Design review of the part built by this model. Coordinates are the model's own, in mm. Face numbers are marked on the shaded views. A direction names the side the tool comes from. Give positions to 0.01 mm unless a question says otherwise; leave off trailing zeros. Loops run counter-clockwise (first coordinate to the right, second up) from the corner with the lowest first, then second, coordinate; pieces in that order, holes last. Notation, with made-up numbers: M 66,61 L 117,61 A25 cw 117,78 Z; hole C 41,81.25 d9. An arc over 180 degrees is marked long. Answer as CSV lines item,"result".
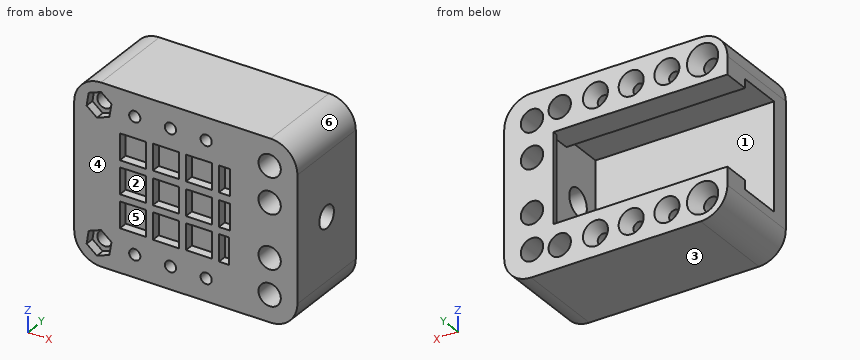
```python
from build123d import *

# Parameters (mm, degrees)
SKETCH1_W                                         = 63.5
SKETCH1_H                                         = 50.8
BOSS_EXTRUDE1_DEPTH                               = 25.4
FILLET1_R                                         = 7.62
CUT_EXTRUDE1_DEPTH                                = 50.8
SKETCH4_W                                         = 49.53
SKETCH4_H                                         = 25.4
CUT_EXTRUDE2_DEPTH                                = 13.462
CSK_FOR_2_FLAT_HEAD_MACHINE_SCREW_100_D           = 4.318
CSK_FOR_2_FLAT_HEAD_MACHINE_SCREW_100_CSINK_D     = 8.89
CSK_FOR_2_FLAT_HEAD_MACHINE_SCREW_100_CSINK_ANGLE = 60
CSK_FOR_2_FLAT_HEAD_MACHINE_SCREW_2_D             = 3.175
CSK_FOR_2_FLAT_HEAD_MACHINE_SCREW_2_CSINK_D       = 7.112
CSK_FOR_2_FLAT_HEAD_MACHINE_SCREW_2_CSINK_ANGLE   = 60
SKETCH9_R                                         = 3.175
CUT_EXTRUDE3_DEPTH                                = 12.7
F_1_4_0_25_DIAMETER_HOLE1_D                       = 6.35
F_1_4_0_25_DIAMETER_HOLE2_D                       = 6.35
CUT_EXTRUDE4_DEPTH                                = 2.54
SKETCH15_W                                        = 3.09588561
SKETCH15_H                                        = 7.430125466
SKETCH15_W_2                                      = 7.430125466
SKETCH15_H_2                                      = 7.430125465
SKETCH15_W_3                                      = 2.91808561
SKETCH15_H_3                                      = 7.607925465
CUT_EXTRUDE5_DEPTH                                = 2.54
SKETCH16_R                                        = 3.175
CUT_EXTRUDE8_DEPTH                                = 6.985
SKETCH17_R                                        = 3.81
CUT_EXTRUDE9_DEPTH                                = 6.985


with BuildPart() as part:
    # Sketch1 → Boss-Extrude1 (new body)
    with BuildSketch(Plane(origin=(0, 0, 0), x_dir=(1, 0, 0), z_dir=(0, 1, 0))):
        with Locations((31.75, 25.4)):
            Rectangle(SKETCH1_W, SKETCH1_H)
    extrude(amount=BOSS_EXTRUDE1_DEPTH)

    # Fillet1
    fillet1_edges = [part.edges().sort_by_distance(p)[0] for p in [
        (0, 12.7, -50.8),
        (63.5, 12.7, -50.8),
        (63.5, 12.7, 0),
        (0, 12.7, 0),
    ]]
    fillet(fillet1_edges, radius=FILLET1_R)

    # Sketch2 → Cut-Extrude1 (cut)
    with BuildSketch(Plane.ZY):
        Polygon((-38.1, 24.003), (-12.7, 24.003), (-12.7, 17.78), (-10.16, 17.78), (-10.16, 5.08), (-40.64, 5.08), (-40.64, 17.78), (-38.1, 17.78), align=None)
    extrude(amount=-CUT_EXTRUDE1_DEPTH, mode=Mode.SUBTRACT)

    # Sketch4 → Cut-Extrude2 (cut)
    with BuildSketch(Plane(origin=(0, 25.4, 0), x_dir=(1, 0, 0), z_dir=(0, 1, 0))):
        with Locations((24.765, 25.4)):
            Rectangle(SKETCH4_W, SKETCH4_H)
    extrude(amount=-CUT_EXTRUDE2_DEPTH, mode=Mode.SUBTRACT)

    # CSK for _2 Flat Head Machine Screw _100 (through all)
    with Locations(Plane(origin=(0, 25.4, 0), x_dir=(1, 0, 0), z_dir=(0, 1, 0))):
        with Locations((7.0612, 44.45)):
            csk_for_2_flat_head_machine_screw_100 = CounterSinkHole(CSK_FOR_2_FLAT_HEAD_MACHINE_SCREW_100_D / 2, CSK_FOR_2_FLAT_HEAD_MACHINE_SCREW_100_CSINK_D / 2, counter_sink_angle=CSK_FOR_2_FLAT_HEAD_MACHINE_SCREW_100_CSINK_ANGLE)

    # CSK for _2 Flat Head Machine Screw _ 2 (through all)
    with Locations(Plane(origin=(0, 25.4, 0), x_dir=(1, 0, 0), z_dir=(0, 1, 0))):
        with Locations((17.2212, 44.45), (27.3812, 44.45), (37.5412, 44.45)):
            csk_for_2_flat_head_machine_screw_2 = CounterSinkHole(CSK_FOR_2_FLAT_HEAD_MACHINE_SCREW_2_D / 2, CSK_FOR_2_FLAT_HEAD_MACHINE_SCREW_2_CSINK_D / 2, counter_sink_angle=CSK_FOR_2_FLAT_HEAD_MACHINE_SCREW_2_CSINK_ANGLE)

    # Sketch9 → Cut-Extrude3 (cut)
    with BuildSketch(Plane(origin=(0, 25.4, 0), x_dir=(1, 0, 0), z_dir=(0, 1, 0))):
        with Locations(Location((47.7012, 44.45, 0), (0, 0, 270))):
            Circle(SKETCH9_R)
    cut_extrude3 = extrude(amount=-CUT_EXTRUDE3_DEPTH, mode=Mode.SUBTRACT)

    # 1/4 (0.25) Diameter Hole1 (through all)
    with Locations(Plane(origin=(0, 25.4, 0), x_dir=(1, 0, 0), z_dir=(0, 1, 0))):
        with Locations((55.6006, 43.18)):
            f_1_4_0_25_diameter_hole1 = Hole(F_1_4_0_25_DIAMETER_HOLE1_D / 2)

    # Mirror1: CSK for _2 Flat Head Machine Screw _100, CSK for _2 Flat Head Machine Screw _ 2, Cut-Extrude3, 1/4 (0.25) Diameter Hole1 across plane
    add(csk_for_2_flat_head_machine_screw_100.mirror(Plane.XY.offset(-25.4)), mode=Mode.SUBTRACT)
    add(csk_for_2_flat_head_machine_screw_2.mirror(Plane.XY.offset(-25.4)), mode=Mode.SUBTRACT)
    add(cut_extrude3.mirror(Plane.XY.offset(-25.4)), mode=Mode.SUBTRACT)
    add(f_1_4_0_25_diameter_hole1.mirror(Plane.XY.offset(-25.4)), mode=Mode.SUBTRACT)

    # 1/4 (0.25) Diameter Hole2 (through all)
    with Locations(Plane(origin=(0, 25.4, 0), x_dir=(1, 0, 0), z_dir=(0, 1, 0))):
        with Locations((55.6006, 33.02), (55.6006, 17.78)):
            Hole(F_1_4_0_25_DIAMETER_HOLE2_D / 2)

    # Sketch14 → Cut-Extrude4 (cut)
    with BuildSketch(Plane.XZ):
        Polygon((9.997746715, -8.735687211), (10.595539088, -4.999719551), (7.658992373, -2.61403234), (4.124653285, -3.964312789), (3.526860912, -7.700280449), (6.463407627, -10.08596766), align=None)
        Polygon((7.658992373, -40.71403234), (4.124653285, -42.064312789), (3.526860912, -45.800280449), (6.463407627, -48.18596766), (9.997746715, -46.835687211), (10.595539088, -43.099719551), align=None)
    extrude(amount=-CUT_EXTRUDE4_DEPTH, mode=Mode.SUBTRACT)

    # Sketch15 → Cut-Extrude5 (cut)
    with BuildSketch(Plane.XZ):
        with Locations((42.72716817, -25.4)):
            Rectangle(SKETCH15_W, SKETCH15_H)
        with Locations((35.508362632, -25.4)):
            Rectangle(SKETCH15_W_2, SKETCH15_H)
        with Locations((26.110362632, -25.4)):
            Rectangle(SKETCH15_W_2, SKETCH15_H)
        with Locations((16.712362632, -25.4)):
            Rectangle(SKETCH15_W_2, SKETCH15_H)
        with Locations((42.72716817, -15.840689934)):
            Rectangle(SKETCH15_W, SKETCH15_H)
        with Locations((16.712362632, -16.014074535)):
            Rectangle(SKETCH15_W_2, SKETCH15_H_2)
        with Locations((35.508362632, -15.840689934)):
            Rectangle(SKETCH15_W_2, SKETCH15_H)
        with Locations((26.110362632, -15.840689934)):
            Rectangle(SKETCH15_W_2, SKETCH15_H)
        with Locations((35.508362632, -34.785925466)):
            Rectangle(SKETCH15_W_2, SKETCH15_H_2)
        with Locations((42.63826817, -34.874825466)):
            Rectangle(SKETCH15_W_3, SKETCH15_H_3)
        with Locations((26.110362632, -34.874825466)):
            Rectangle(SKETCH15_W_2, SKETCH15_H_3)
        with Locations((16.712362632, -34.785925466)):
            Rectangle(SKETCH15_W_2, SKETCH15_H_2)
    extrude(amount=-CUT_EXTRUDE5_DEPTH, mode=Mode.SUBTRACT)

    # Sketch16 → Cut-Extrude8 (cut)
    with BuildSketch(Plane(origin=(63.5, 0, 0), x_dir=(0, 0, -1), z_dir=(1, 0, 0))):
        with Locations((25.4, 12.7)):
            Circle(SKETCH16_R)
    extrude(amount=-CUT_EXTRUDE8_DEPTH, mode=Mode.SUBTRACT)

    # Sketch17 → Cut-Extrude9 (cut)
    with BuildSketch(Plane.ZY.offset(-50.8)):
        with Locations((-25.4, 12.7)):
            Circle(SKETCH17_R)
    extrude(amount=-CUT_EXTRUDE9_DEPTH, mode=Mode.SUBTRACT)


solid = part.part
```
1. For P1, Ø1.5, axis at y = 25, z = -28, coming from the -X side; P2, Ø6, axis at x = 15.5, z = -16.5, coming from the +Y side; P3, Ø3.5, axis at x = 36.5, z = -25, coming from the -Y side, all flat-tipped, find the tip position at first contact; note any pin that passes through.
Answer block:
P1,"x = 49.53"
P2,"y = 5.08"
P3,"y = 2.54"
2. The part is to be moulded in two halves that separate along X. For the marked faces 4, 5 and 6, say which applies: pulls with the +X half, pulls with the -X half, needs draft (parallel to the pull), parting line crosses it, or undercut.
Answer block:
face 4,"needs draft"
face 5,"undercut"
face 6,"pulls with the +X half"
3. We need section D-D, the plane z = -17.78. Write out the cut boundary in (x, y).
Answer block:
outline,"M 0,0 L 13,0 L 13,2.54 L 20.43,2.54 L 20.43,0 L 22.4,0 L 22.4,2.54 L 29.83,2.54 L 29.83,0 L 31.79,0 L 31.79,2.54 L 39.22,2.54 L 39.22,0 L 41.18,0 L 41.18,2.54 L 44.28,2.54 L 44.28,0 L 52.43,0 L 52.43,25.4 L 49.53,25.4 L 49.53,24 L 50.8,24 L 50.8,5.08 L 0,5.08 Z; M 58.78,0 L 63.5,0 L 63.5,25.4 L 58.78,25.4 Z"
4. We need section C-C, the plane z = -44.45. Count the separate pieces of the cut face and the enclosed holes in it, plus the area to 3 significant figures.
Answer block:
separate pieces,"6"
enclosed holes,"0"
area,"992 mm²"
5. We need section A-A, the plane z = -33.02. Write out the cut boundary in (x, y), plus the area to 3 significant figures.
Answer block:
outline,"M 0,0 L 13,0 L 13,2.54 L 20.43,2.54 L 20.43,0 L 22.4,0 L 22.4,2.54 L 29.83,2.54 L 29.83,0 L 31.79,0 L 31.79,2.54 L 39.22,2.54 L 39.22,0 L 41.18,0 L 41.18,2.54 L 44.1,2.54 L 44.1,0 L 52.43,0 L 52.43,25.4 L 49.53,25.4 L 49.53,24 L 50.8,24 L 50.8,5.08 L 0,5.08 Z; M 58.78,0 L 63.5,0 L 63.5,25.4 L 58.78,25.4 Z"
area,"357 mm²"
6. To check wall thickness, follow L1, parallel to Z at x = 24.5, y = 11.5; L2, parallel to Z at x = 43, y = 21; L3, parallel to Z at x = 37.5, y = 12.25. State the ranges of each line that lie inside material, in increasing order. Write a range as [from, to].
Answer block:
L1,"[-50.8, -40.64], [-10.16, 0]"
L2,"[-50.8, -38.1], [-12.7, 0]"
L3,"[-50.8, -46.04], [-42.86, -40.64], [-10.16, -7.94], [-4.76, 0]"
7. For the marked faces 1, 2 and 3, list the 3-axis set-ups (+Z, -Z, +X, -X, +Y, -Y) from which the entire face can be reached by the end or side of a thin tool; tool diameter is ignored.
Answer block:
face 1,"-X"
face 2,"-Y"
face 3,"-Z, +X, -X, +Y, -Y"
